```python
from build123d import *

# Parameters (mm, degrees)
SKETCH1_W            = 80.762
SKETCH1_H            = 75.312
BOSS_EXTRUDE1_DEPTH  = 50
SHELL1_T             = 4
M4_CLEARANCE_HOLE1_D = 4.8


with BuildPart() as part:
    # Sketch1 → Boss-Extrude1 (new body)
    with BuildSketch(Plane.XY):
        Rectangle(SKETCH1_W, SKETCH1_H)
    extrude(amount=BOSS_EXTRUDE1_DEPTH)

    # Shell1
    shell1_openings = [part.faces().sort_by_distance(p)[0] for p in [
        (0, 0, 50),
    ]]
    offset(amount=SHELL1_T, openings=shell1_openings, kind=Kind.INTERSECTION)

    # M4 Clearance Hole1 (through all)
    with Locations(Plane(origin=(44.381, 0, 0), x_dir=(0, 0, -1), z_dir=(1, 0, 0))):
        with Locations((-33.35, -17.5), (-6.35, -17.5), (-33.35, 17.5), (-6.35, 17.5)):
            Hole(M4_CLEARANCE_HOLE1_D / 2)


solid = part.part
```
Work out the finished part from the listing and answer in its coordinate system (mm). A direction names the side the tool comes from. Coordinates: 2 decimals unless noted, no trailing zeros. Order: outer loops, then holes, each group sorted by start corner. A loop starts at its lowest first (then second) coordinate and runs counter-clockwise, first axis right, second up. Notation, with made-up numbers: M -0.75,66 L 57.25,66 A14 cw 57.25,90 Z; hole C 41.25,28.5 d2. An arc over 180 degrees is marked long. Use CSV: the item, a comma, the result in double quotes.
1) Section D-D on x = 13 is taken. Write down the section's boundary in (y, z).
Worked out:
outline,"M -41.66,-4 L 41.66,-4 L 41.66,50 L 37.66,50 L 37.66,0 L -37.66,0 L -37.66,50 L -41.66,50 Z"
2) Section C-C on z = 18.5 is taken. Write down the section's boundary in (x, y), plus the area to 3 significant figures.
Worked out:
outline,"M -44.38,-41.66 L 44.38,-41.66 L 44.38,41.66 L -44.38,41.66 Z; hole M -40.38,-37.66 L 40.38,-37.66 L 40.38,37.66 L -40.38,37.66 Z"
area,"1,310 mm^2"
3) Determine the mould class of faces 3 (the face through (-1, 1, -4)), 4 (the face through (44.381, -1, 23)), 5 (the face through (-40.381, -1, 25)) for opening direction X: released by +X, released by -X, zero draft, split by the parting line, or undercut.
Worked out:
face 3,"zero draft"
face 4,"released by +X"
face 5,"undercut"
4) Section B-B on z = 33.35 is taken. Write down the section's boundary in (x, y), plus the area to 3 significant figures.
Worked out:
outline,"M -44.38,-41.66 L 44.38,-41.66 L 44.38,-19.9 L 40.38,-19.9 L 40.38,-37.66 L -40.38,-37.66 L -40.38,-19.9 L -44.38,-19.9 Z; M -44.38,-15.1 L -40.38,-15.1 L -40.38,15.1 L -44.38,15.1 Z; M -44.38,19.9 L -40.38,19.9 L -40.38,37.66 L 40.38,37.66 L 40.38,19.9 L 44.38,19.9 L 44.38,41.66 L -44.38,41.66 Z; M 40.38,-15.1 L 44.38,-15.1 L 44.38,15.1 L 40.38,15.1 Z"
area,"1,240 mm^2"
5) Section A-A on y = 17.5 is taken. Write down the section's boundary in (x, z), plus the area to 3 significant figures.
Worked out:
outline,"M -44.38,-4 L 44.38,-4 L 44.38,3.95 L 40.38,3.95 L 40.38,0 L -40.38,0 L -40.38,3.95 L -44.38,3.95 Z; M -44.38,8.75 L -40.38,8.75 L -40.38,30.95 L -44.38,30.95 Z; M -44.38,35.75 L -40.38,35.75 L -40.38,50 L -44.38,50 Z; M 40.38,8.75 L 44.38,8.75 L 44.38,30.95 L 40.38,30.95 Z; M 40.38,35.75 L 44.38,35.75 L 44.38,50 L 40.38,50 Z"
area,"678 mm^2"
6) A flat-ended cylindrical pin translates along its axis: pin 1 Ø2 at (x, y) = (-25.5, -24.5) entering from +Z. Find the tip coordinate at first contact, or state that the pin passes through.
Worked out:
pin 1,"stops at z = 0"
7) Consider line 1 (X direction, y = 29, z = 34.5); line 2 (Y direction, x = -29, z = 2); line 3 (Y direction, x = -42.85, z = 6.35). Determine where each line is inside the solid, lowest interval first. Write a range as [from, to].
Worked out:
line 1,"x = [-44.38, -40.38], [40.38, 44.38]"
line 2,"y = [-41.66, -37.66], [37.66, 41.66]"
line 3,"y = [-41.66, -19.9], [-15.1, 15.1], [19.9, 41.66]"
8) For faces 1 (the face through (-3, -40, 50)), 2 (the face through (-1, 1, 0)), determine the directions among +Z, -Z, +X, -X, +Y, -Y from which every point of the face is accessible in a straight line to the end or side of a thin tool.
Worked out:
face 1,"+Z, +X, -X, +Y, -Y"
face 2,"+Z"
